Geometry check sheet. Reference: drawing and pictorial views, mm from the part's lowest x, y, z. A direction names the side the tool comes from. Give positions to 0.01 mm unless a question says otherwise; leave off trailing zeros. Write each loop counter-clockwise with the first axis right and the second up, starting at its lowest first coordinate (ties: lowest second). Pieces come first, ordered by that corner, then holes. Notation, with made-up numbers: (31.5, 70.25) -> (69.5, 70.25) arc R17 cw to (69.5, 76.25) -> close; hole circle Ø10 at (69.5, 42.25). An arc over 180 degrees is marked (long way). Return JSON: item names as keys, results as strings.
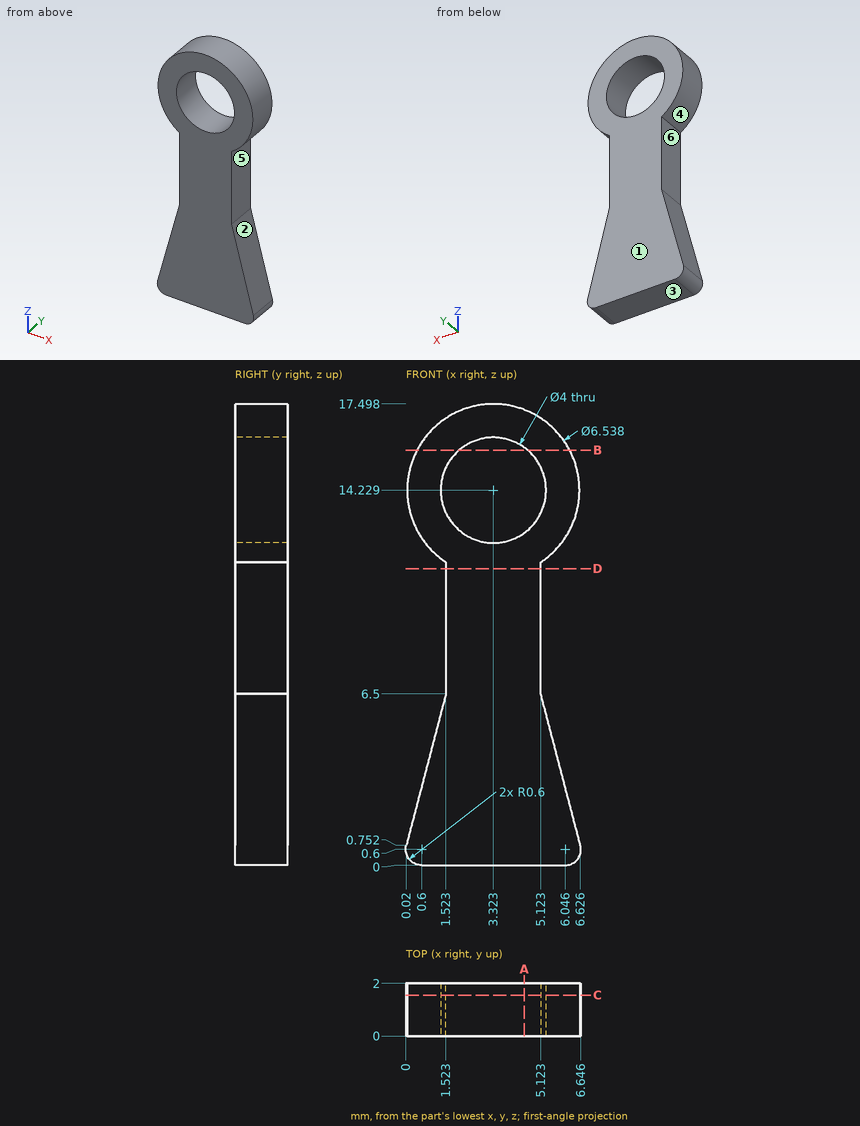
(1) Thickness scan on L1, parallel to X at y = 1.25, z = 14.25; L2, parallel to X at y = 1.55, z = 11; L3, parallel to X at y = 0.6, z = 15.25 (1 decimal). Record the ranges inside material, lowest first.
Reply:
{"L1": "0.05 to 1.32, 5.32 to 6.59", "L2": "1.52 to 5.12", "L3": "0.2 to 1.6, 5 to 6.4"}
(2) Cross-section at C-C on y = 1.55. Enter the section's corners in (x, z) (1 decimal).
Reply:
{"outline": "(0, 0.8) arc R0.6 ccw to (0.6, 0) -> (6, 0) arc R0.6 ccw to (6.6, 0.8) -> (5.1, 6.5) -> (5.1, 11.5) arc R3.3 ccw (long way) to (1.5, 11.5) -> (1.5, 6.5) -> close; hole circle Ø4 at (3.3, 14.2)"}
(3) Set-up check for the marked faces 4, 5 and 6: record each of +Z, -Z, +X, -X, +Y, -Y from which the full face is reachable in a straight line by a thin tool's end or side.
Reply:
{"face 4": "+Y, -Y", "face 5": "+X, +Y, -Y", "face 6": "-X, +Y, -Y"}
(4) Release check for a two-part mould opening along Z. For the marked faces 1, 2 and 3 record: pulls with the +Z half, pulls with the -Z half, needs draft (parallel to the pull), parting line crosses it, or undercut.
Reply:
{"face 1": "needs draft", "face 2": "undercut", "face 3": "pulls with the -Z half"}
(5) Cross-section at B-B on z = 15.75. Enter the section's corners in (x, y) (1 decimal).
Reply:
{"outline": "(0.4, 0) -> (2, 0) -> (2, 2) -> (0.4, 2) -> close; (4.6, 0) -> (6.2, 0) -> (6.2, 2) -> (4.6, 2) -> close"}
(6) Cross-section at A-A on x = 4.5. Enter the section's corners in (y, z) (1 decimal).
Reply:
{"outline": "(0, 0) -> (2, 0) -> (2, 12.6) -> (0, 12.6) -> close; (0, 15.8) -> (2, 15.8) -> (2, 17.3) -> (0, 17.3) -> close"}
(7) Cross-section at D-D on z = 11.25. Enter the section's corners in (x, y).
Reply:
{"outline": "(1.52, 0) -> (5.12, 0) -> (5.12, 2) -> (1.52, 2) -> close"}
